```python
from build123d import *

# Parameters (mm, degrees)
DISCO_START    = 3.175
CROQUIS5_R     = 15
DISCO_DEPTH    = 5.67
BARRENOS_START = 3.175
CROQUIS6_R     = 1.7
CROQUIS6_R_2   = 2.05
CROQUIS6_R_3   = 4.5
BARRENOS_DEPTH = 5.67


with BuildPart() as part:
    # Croquis5 → Disco (new body)
    with BuildSketch(Plane(origin=(0, 0, 0), x_dir=(1, 0, 0), z_dir=(0, 1, 0)).offset(DISCO_START)):
        with Locations(Location((152.4, -171.45, 0), (0, 0, 270))):
            Circle(CROQUIS5_R)
    extrude(amount=DISCO_DEPTH)

    # Croquis6 → Barrenos (cut)
    with BuildSketch(Plane(origin=(0, 0, 0), x_dir=(1, 0, 0), z_dir=(0, 1, 0)).offset(BARRENOS_START)):
        with Locations(Location((163.416293151, -177.356884561, 0), (0, 0, 270))):
            Circle(CROQUIS6_R)
        with Locations(Location((152.792634488, -183.943832005, 0), (0, 0, 270))):
            Circle(CROQUIS6_R)
        with Locations(Location((141.776341338, -178.036947444, 0), (0, 0, 270))):
            Circle(CROQUIS6_R)
        with Locations(Location((141.383706849, -165.543115439, 0), (0, 0, 270))):
            Circle(CROQUIS6_R)
        with Locations(Location((152.007365512, -158.956167995, 0), (0, 0, 270))):
            Circle(CROQUIS6_R)
        with Locations(Location((163.023658662, -164.863052556, 0), (0, 0, 270))):
            Circle(CROQUIS6_R)
        with Locations(Location((157.774949114, -180.118905468, 0), (0, 0, 270))):
            Circle(CROQUIS6_R_2)
        with Locations(Location((142.205033084, -171.770389743, 0), (0, 0, 270))):
            Circle(CROQUIS6_R_2)
        with Locations(Location((157.220017802, -162.460704789, 0), (0, 0, 270))):
            Circle(CROQUIS6_R_2)
        with Locations(Location((152.4, -171.45, 0), (0, 0, 270))):
            Circle(CROQUIS6_R_3)
    extrude(amount=BARRENOS_DEPTH, mode=Mode.SUBTRACT)


solid = part.part
```
Input: part model. Units: mm. Frame: model coordinates. Round coordinates to 2 decimals unless told otherwise and drop trailing zeros. Loops run counter-clockwise (first coordinate to the right, second up) from the corner with the lowest first, then second, coordinate; pieces in that order, holes last. Notation, with made-up numbers: (82.5, 6.5) -> (120.5, 6.5) arc R15 cw to (120.5, 20.5) -> close; hole circle Ø2 at (69, 53). An arc over 180 degrees is marked (long way). Use one line per item in the form item = value. Start each with the question number.
Item 1: Section query D-D on x = 148.75. Return the cut outline in (y, z) (3 decimals).
Item 2: Material intervals for L1, parallel to X at y = 6.9, z = 164.75; L2, parallel to Z at x = 156.25, y = 6.5; L3, parallel to Z at x = 153.5, y = 4.55, sorted ascending. Write a range as from..to.
Item 3: Mould query, pull axis Z, two halves, no side actions, for faces 1 (the face through (156, 8.845, 175)), 2 (the face through (159.504, 5.97, 181.221)), 3 (the face through (156.906, 5.97, 185.757)), 4 (the face through (153.44, 5.97, 159.87)). Classes: pulls with the +Z half, pulls with the -Z half, needs draft (parallel to the pull), parting line crosses it, or undercut.
Item 4: Section query B-B on y = 7.5. Count the separate pieces of the cut face and the enclosed holes in it, then the cut area to 3 significant figures.
Item 5: Section query A-A on x = 140.75. Return the cut outline in (y, z) (3 decimals).
Item 6: Contact query for flat-ended pins moving along their axis: pin 1 Ø1.5 at (x, y) = (151, 7) entering from -Z; pin 2 Ø1.5 at (y, z) = (5.5, 181) entering from -X; pin 3 Ø3 at (x, z) = (141.38, 165.54) entering from -Y; pin 4 Ø2 at (y, z) = (6, 183.5) entering from +X. Output: stop coordinate, or through.
Item 7: Section query C-C on z = 168.5. Return the cut outline in (x, y) (3 decimals), then the cut area to 3 significant figures.
Ans:
q1.outline = (3.175, 156.901) -> (8.845, 156.901) -> (8.845, 168.818) -> (3.175, 168.818) -> close; (3.175, 174.082) -> (8.845, 174.082) -> (8.845, 185.999) -> (3.175, 185.999) -> close
q2.L1 = 138.98..139.88, 142.89..161.33, 164.72..165.82
q2.L2 = 156.95..160.65, 164.27..169.12, 173.78..178.75, 181.49..185.95
q2.L3 = 156.49..158.14, 159.77..167.09, 175.81..182.4, 185.49..186.41
q3.face_1 = needs draft
q3.face_2 = undercut
q3.face_3 = parting line crosses it
q3.face_4 = undercut
q4.separate_pieces = 1
q4.enclosed_holes = 10
q4.area = 549 mm^2
q5.outline = (3.175, 162.001) -> (8.845, 162.001) -> (8.845, 163.966) -> (3.175, 163.966) -> close; (3.175, 167.121) -> (8.845, 167.121) -> (8.845, 170.326) -> (3.175, 170.326) -> close; (3.175, 173.214) -> (8.845, 173.214) -> (8.845, 176.682) -> (3.175, 176.682) -> close; (3.175, 179.392) -> (8.845, 179.392) -> (8.845, 180.899) -> (3.175, 180.899) -> close
q6.pin_1 = 156.46
q6.pin_2 = 140.25
q6.pin_3 = through
q6.pin_4 = 162.54
q7.outline = (137.693, 3.175) -> (149.002, 3.175) -> (149.002, 8.845) -> (137.693, 8.845) -> close; (155.798, 3.175) -> (167.107, 3.175) -> (167.107, 8.845) -> (155.798, 8.845) -> close
q7.area = 128 mm^2
